Design review of the part built by this model. Coordinates are the model's own, in mm. A direction names the side the tool comes from. Round coordinates to 2 decimals unless told otherwise and drop trailing zeros. Write each loop counter-clockwise with the first axis right and the second up, starting at its lowest first coordinate (ties: lowest second). Pieces come first, ordered by that corner, then holes. Notation, with made-up numbers: (77.5, 11.25) - (99.5, 11.25) arc R25 cw to (99.5, 32.25) - close; hole circle Ø4 at (-15, 80.25). An arc over 180 degrees is marked (long way). Use one line per item in the form item = value.
```python
from build123d import *

# Parameters (mm, degrees)
SKETCH1_R           = 6
SKETCH1_R_2         = 3
SKETCH1_R_3         = 1.5
SKETCH1_R_4         = 1.25
SKETCH1_W           = 8
SKETCH1_H           = 2.4
BOSS_EXTRUDE1_DEPTH = 5
SKETCH2_R           = 1.2
CUT_EXTRUDE1_DEPTH  = 6


with BuildPart() as part:
    # Sketch1 → Boss-Extrude1 (new body)
    with BuildSketch(Plane(origin=(0, 0, 0), x_dir=(0, 0, -1), z_dir=(1, 0, 0))):
        Polygon((0, 0), (-50, 0), (-50, 25), (-55, 25), (-55, 40), (-50, 40), (-50, 47), (-45, 47), (-45, 53), (-50, 53), (-50, 64), (0, 64), (0, 49), (-5, 49), (-5, 24), (0, 24), align=None)
        with Locations((-20, 17)):
            Circle(SKETCH1_R, mode=Mode.SUBTRACT)
        with Locations((-25, 44)):
            Circle(SKETCH1_R_2, mode=Mode.SUBTRACT)
        with Locations((-45, 7.5)):
            Circle(SKETCH1_R_3, mode=Mode.SUBTRACT)
        with Locations((-38, 57)):
            Circle(SKETCH1_R_4, mode=Mode.SUBTRACT)
        with Locations((-12, 57)):
            Circle(SKETCH1_R_4, mode=Mode.SUBTRACT)
        with Locations((-38, 31)):
            Circle(SKETCH1_R_4, mode=Mode.SUBTRACT)
        with Locations((-12, 31)):
            Circle(SKETCH1_R_4, mode=Mode.SUBTRACT)
        with Locations((-32, 7.5)):
            Circle(SKETCH1_R_3, mode=Mode.SUBTRACT)
        with Locations((-38.5, 18.2)):
            Rectangle(SKETCH1_W, SKETCH1_H, mode=Mode.SUBTRACT)
    extrude(amount=BOSS_EXTRUDE1_DEPTH)

    # Sketch2 → Cut-Extrude1 (cut, through all)
    with BuildSketch(Plane.ZY):
        with Locations((2.5, 56.5)):
            Circle(SKETCH2_R)
        with Locations((2.5, 12)):
            Circle(SKETCH2_R)
        Polygon((50, 59.7), (46, 59.7), (46, 61.25), (44.2, 61.25), (44.2, 59.7), (42.2, 59.7), (42.2, 57.3), (44.2, 57.3), (44.2, 55.75), (46, 55.75), (46, 57.3), (50, 57.3), align=None)
        Polygon((50, 19.4), (46, 19.4), (46, 20.95), (44.2, 20.95), (44.2, 19.4), (42.2, 19.4), (42.2, 17), (44.2, 17), (44.2, 15.45), (46, 15.45), (46, 17), (50, 17), align=None)
    extrude(amount=-CUT_EXTRUDE1_DEPTH, mode=Mode.SUBTRACT)


solid = part.part
```
Q1. We need section D-D on z = 17. Write out the cut boundary in (x, y), then the cut area to 3 significant figures.
Calculated:
outline = (0, 0) - (5, 0) - (5, 11.8) - (0, 11.8) - close; (0, 22.2) - (5, 22.2) - (5, 64) - (0, 64) - close
area = 268 mm2
Q2. Machinability: for faces 4 (the flat face through (2, 57, 44.2)), 5 (the flat face through (2, 22, 50)), 6 (the flat face through (2, 55, 50)), which of the approach directions +Z, -Z, +X, -X, +Y, -Y give a long, thin tool a straight path to every point of the face, cutting with its end or side? Answer none if there is none.
Calculated:
face_4 = +X, -X
face_5 = +Z, +X, -X, -Y
face_6 = +Z, +X, -X, +Y
Q3. For P1, Ø2, axis at x = 2.5, z = 18, coming from the -Y side; P2, Ø1.9, axis at x = 2.5, y = 58, coming from the +Z side; P3, Ø5, axis at y = 44, z = 25, coming from the +X side, all flat-tipped, find the tip position at first contact; note any pin that passes through.
Calculated:
P1 = 0
P2 = 50
P3 = through
Q4. We need section C-C on y = 14. Write out the cut boundary in (x, z).
Calculated:
outline = (0, 0) - (5, 0) - (5, 14.8) - (0, 14.8) - close; (0, 25.2) - (5, 25.2) - (5, 50) - (0, 50) - close
Q5. Draft analysis for pull direction Z (two halves, no side actions). For faces 1 (the flat face through (5, 32, 27)), 2 (the cylindrical face through (2.46, 13.35, 24.76)), 3 (the flat face through (2, 62, 50)), state which applies: released by +Z, released by -Z, zero draft, split by the parting line, or undercut.
Calculated:
face_1 = zero draft
face_2 = undercut
face_3 = released by +Z
Q6. We need section A-A on z = 47.5. Write out the cut boundary in (x, y).
Calculated:
outline = (0, 0) - (5, 0) - (5, 17) - (0, 17) - close; (0, 19.4) - (5, 19.4) - (5, 47) - (0, 47) - close; (0, 53) - (5, 53) - (5, 57.3) - (0, 57.3) - close; (0, 59.7) - (5, 59.7) - (5, 64) - (0, 64) - close
Q7. We need section B-B on y = 7.5. Write out the cut boundary in (x, z).
Calculated:
outline = (0, 0) - (5, 0) - (5, 30.5) - (0, 30.5) - close; (0, 33.5) - (5, 33.5) - (5, 43.5) - (0, 43.5) - close; (0, 46.5) - (5, 46.5) - (5, 50) - (0, 50) - close
Q8. To check wall thickness, follow line 1 along Y through (x, z) = (2.3, 47); line 2 along Y through (x, z) = (3.1, 2.5); line 3 along Y through (x, z) = (1, 42.5). State the ranges of each line that lie inside material, in increasing order. Write a range as from..to.
Calculated:
line_1 = 0..17, 19.4..47, 53..57.3, 59.7..64
line_2 = 0..10.8, 13.2..24, 49..55.3, 57.7..64
line_3 = 0..17, 19.4..57.3, 59.7..64
